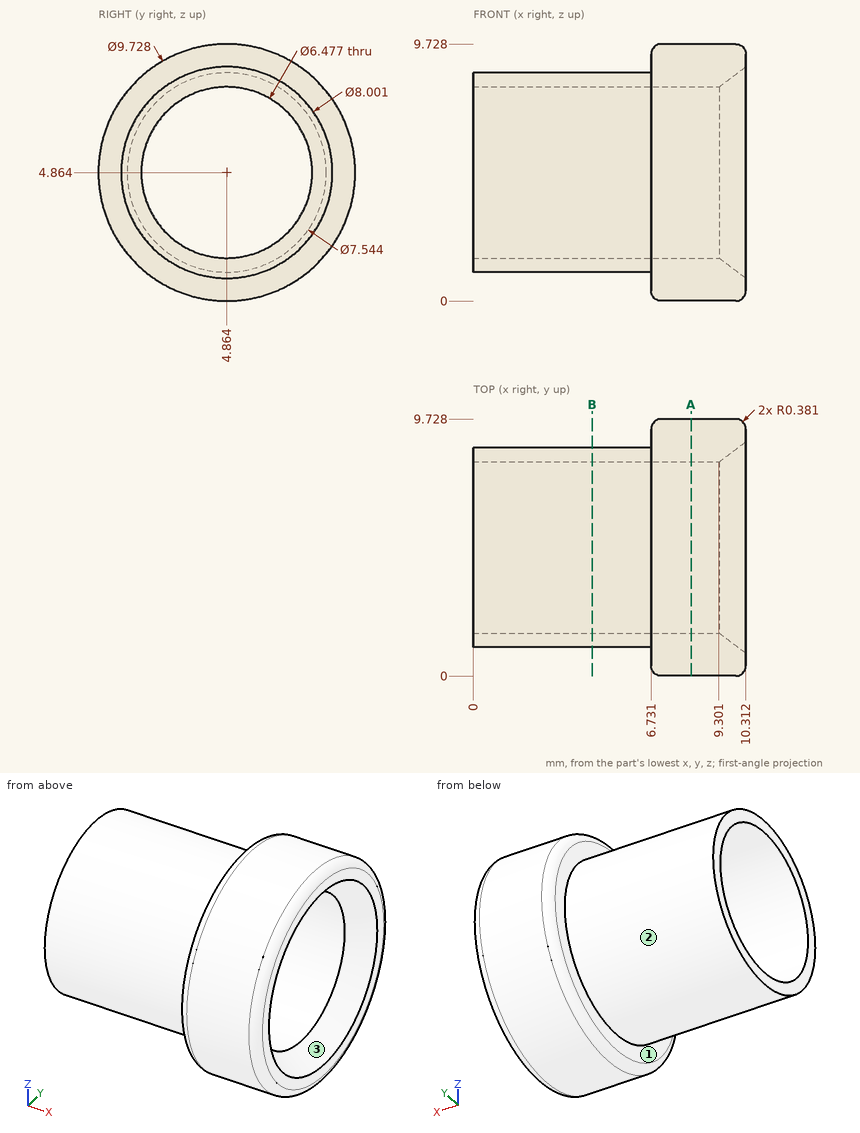
Check sheet for the drawn part. Datum: minimum x, y, z corner. Units: mm. Round coordinates to 2 decimals unless told otherwise and drop trailing zeros. Write each loop counter-clockwise with the first axis right and the second up, starting at its lowest first coordinate (ties: lowest second). Pieces come first, ordered by that corner, then holes. Notation, with made-up numbers: (18, 26.25) -> (71, 26.25) arc R27 ccw to (71, 63.25) -> close; hole circle Ø4 at (28, -8). An arc over 180 degrees is marked (long way). Put each result on its own line as item: value.
(1) Go/stop test with flat-tipped pins: pin 1 Ø4 at (x, z) = (5.5, 3) entering from -Y; pin 2 Ø1 at (x, z) = (4, 5) entering from +Y; pin 3 Ø2.5 at (y, z) = (4.5, 4) entering from -X. Record where each tip stops, or that it passes through.
Values found:
pin 1: stops at y = 0.04
pin 2: stops at y = 8.64
pin 3: passes through
(2) Mould release check, pull along Y, two halves, no side actions. Record for the marked faces 1, 2 and 3: released by +Y, released by -Y, zero draft, split by the parting line, or undercut.
Values found:
face 1: zero draft
face 2: split by the parting line
face 3: undercut
(3) Material ranges on line 1 (Y direction, x = 3.5, z = 4.75) (1 decimal); line 2 (X direction, y = 6.5, z = 8.75), recorded low to high.
Values found:
line 1: y = 1.1 to 1.6, 8.1 to 8.6
line 2: x = 6.73 to 10.31
(4) Sectioned sample at B-B (x = 4.5). Enter the section's corners in (y, z).
Values found:
outline: circle Ø7.54 at (4.86, 4.86); hole circle Ø6.48 at (4.86, 4.86)
(5) Sectioned sample at A-A (x = 8.25). Enter the section's corners in (y, z).
Values found:
outline: circle Ø9.73 at (4.86, 4.86); hole circle Ø6.48 at (4.86, 4.86)
